from build123d import *

# Parameters (mm, degrees)
EXTRUDE_1_DEPTH     = 10
SKETCH_2_R          = 5
CUT_EXTRUDE_1_DEPTH = 10
SKETCH_3_R          = 5
CUT_EXTRUDE_2_DEPTH = 10


with BuildPart() as part:
    # 草图1 → 凸台-拉伸1 (new body)
    with BuildSketch(Plane.XY):
        with BuildLine():
            Line((0, -10), (68.35, -10))
            ThreePointArc((68.35, -10), (78.35, 0), (68.35, 10))
            Line((68.35, 10), (0, 10))
            ThreePointArc((0, 10), (-10, 0), (0, -10))
        make_face()
    extrude(amount=EXTRUDE_1_DEPTH)

    # 草图2 → 切除-拉伸1 (cut)
    with BuildSketch(Plane.XY.offset(10)):
        Circle(SKETCH_2_R)
    extrude(amount=-CUT_EXTRUDE_1_DEPTH, mode=Mode.SUBTRACT)

    # 草图3 → 切除-拉伸2 (cut)
    with BuildSketch(Plane.XY.offset(10)):
        with Locations((68.35, 0)):
            Circle(SKETCH_3_R)
    extrude(amount=-CUT_EXTRUDE_2_DEPTH, mode=Mode.SUBTRACT)


solid = part.part
Check sheet for the modelled part. Datum: model origin and axes. Units: mm. Give positions to 0.01 mm unless a question says otherwise; leave off trailing zeros. Loops run counter-clockwise (first coordinate to the right, second up) from the corner with the lowest first, then second, coordinate; pieces in that order, holes last. Notation, with made-up numbers: M -14.75,-12.5 L 4.25,-12.5 A22 cw 4.25,13.5 Z; hole C 74,-19 d4. An arc over 180 degrees is marked long. Return JSON: item names as keys, results as strings. Group by question number.
1. Cross-section at C-C on y = -7.25. Record the boundary of the cut face in (x, z).
2. Go/stop test with flat-tipped pins: pin 1 (3 mm diameter, centred on y = 4, z = 9, fed in from +X); pin 2 (1 mm diameter, centred on x = 58.5, y = -6.5, fed in from -Z); pin 3 (5 mm diameter, centred on y = 4, z = 3, fed in from +X). Record where each tip stops, or that it passes through.
3. Mould release check, pull along X, two halves, no side actions. Record for faces 1 (the flat face through (35, 10, 5)), 2 (the cylindrical face through (72.969, -1.915, 5.07)), 3 (the cylindrical face through (-1.08, -4.88, 5.07)), 4 (the cylindrical face through (-10, 0, 5)): released by +X, released by -X, zero draft, split by the parting line, or undercut.
4. Thickness scan on L1, parallel to Y at x = 0, z = 8; L2, parallel to X at y = 1.5, z = 1.5; L3, parallel to X at y = -2.25, z = 2.5. Record the ranges inside material, lowest first.
5. Cross-section at A-A on y = 0. Record the boundary of the cut face in (x, z), plus the area to 4 significant figures.
6. Cross-section at B-B on z = 4. Record the boundary of the cut face in (x, y).
Return value:
{
 "1": {"outline": "M -6.89,0 L 75.24,0 L 75.24,10 L -6.89,10 Z"},
 "2": {"pin 1": "x = 78.03", "pin 2": "z = 0", "pin 3": "x = 78.24"},
 "3": {"face 1": "zero draft", "face 2": "undercut", "face 3": "undercut", "face 4": "released by -X"},
 "4": {"L1": "-10 to -5, 5 to 10", "L2": "-9.89 to -4.77, 4.77 to 63.58, 73.12 to 78.24", "L3": "-9.74 to -4.47, 4.47 to 63.88, 72.82 to 78.09"},
 "5": {"outline": "M -10,0 L -5,0 L -5,10 L -10,10 Z; M 5,0 L 63.35,0 L 63.35,10 L 5,10 Z; M 73.35,0 L 78.35,0 L 78.35,10 L 73.35,10 Z", "area": "683.5 mm^2"},
 "6": {"outline": "M 0,-10 L 68.35,-10 A10 ccw 68.35,10 L 0,10 A10 ccw Z; hole C 0,0 d10; hole C 68.35,0 d10"}
}
